from build123d import *

# Parameters (mm, degrees)
SKIZZE1_R                       = 4
AUFSATZ_LINEAR_AUSTRAGEN1_DEPTH = 82.5


with BuildPart() as part:
    # Skizze1 → Aufsatz-Linear austragen1 (new, symmetric)
    with BuildSketch(Plane.XY):
        Polygon((-30, 8), (1.899494937, 8), (8.103084379, 1.796410558), (4.537482533, -8), (-3.153212483, -8), (-30, 7.5), align=None)
        Circle(SKIZZE1_R, mode=Mode.SUBTRACT)
    extrude(amount=AUFSATZ_LINEAR_AUSTRAGEN1_DEPTH, both=True)


solid = part.part
Work out the finished part from the listing and answer in its coordinate system (mm). Round coordinates to 2 decimals unless told otherwise and drop trailing zeros. Write each loop counter-clockwise with the first axis right and the second up, starting at its lowest first coordinate (ties: lowest second). Pieces come first, ordered by that corner, then holes.
1) Given pin 1 Ø3 at (y, z) = (-4.5, -44.5) entering from -X; pin 2 Ø5 at (x, z) = (-19, 40) entering from -Y; pin 3 Ø12 at (x, z) = (-19.5, 5.5) entering from -Y, each flat-ended and moving along its own axis, determine where each tip first touches the part or whether it passes through.
2) A cutting plane is placed at D-D (y = -6.5). Give the vertices of the cut face in (x, z).
3) The mould has two halves that part along Y. Classify faces 1 (the flat face through (-6, 2, -82.5)), 2 (the cylindrical face through (-0.867, -3.905, -1.155)), 3 (the flat face through (5, 4.9, 1.2)): pulls with the +Y half, pulls with the -Y half, needs draft (parallel to the pull), parting line crosses it, or undercut.
4) A cutting plane is placed at C-C (y = 0). Give the vertices of the cut face in (x, z), plus the area to 3 significant figures.
5) Straight lines are drawn through the part: line 1 (Y direction, x = 0.5, z = 56); line 2 (X direction, y = 1.5, z = 51.5); line 3 (X direction, y = -2, z = -43). For each, find the intervals that lie inside material, in ascending order.
6) A cutting plane is placed at B-B (z = -22). Give the vertices of the cut face in (x, y).
7) A cutting plane is placed at A-A (x = 0). Give the vertices of the cut face in (y, z), plus the area to 3 significant figures.
Completed:
1. pin 1: stops at x = -11.81
1. pin 2: stops at y = -0.29
1. pin 3: stops at y = -2.03
2. outline: (-5.75, -82.5) - (5.08, -82.5) - (5.08, 82.5) - (-5.75, 82.5) - close
3. face 1: needs draft
3. face 2: undercut
3. face 3: pulls with the +Y half
4. outline: (-17.01, -82.5) - (-4, -82.5) - (-4, 82.5) - (-17.01, 82.5) - close; (4, -82.5) - (7.45, -82.5) - (7.45, 82.5) - (4, 82.5) - close
4. area: 2,720 mm2
5. line 1: y = -8 to -3.97, 3.97 to 8
5. line 2: x = -19.61 to -3.71, 3.71 to 8
5. line 3: x = -13.55 to -3.46, 3.46 to 6.72
6. outline: (-30, 7.5) - (-3.15, -8) - (4.54, -8) - (8.1, 1.8) - (1.9, 8) - (-30, 8) - close; hole circle Ø8 at (0, 0)
7. outline: (-8, -82.5) - (-4, -82.5) - (-4, 82.5) - (-8, 82.5) - close; (4, -82.5) - (8, -82.5) - (8, 82.5) - (4, 82.5) - close
7. area: 1,320 mm2
